Geometry: see drawing. Coordinates: mm, zero at the bounding-box minimum. Give positions to 0.01 mm unless a question says otherwise; leave off trailing zeros. Write each loop counter-clockwise with the first axis right and the second up, starting at its lowest first coordinate (ties: lowest second). Pieces come first, ordered by that corner, then holes. Notation, with made-up numbers: (-16, -25) -> (32, -25) arc R23 cw to (32, -12) -> close; hole circle Ø7 at (-5.5, 26). An arc over 180 degrees is marked (long way). Use one line per item in the form item = value. Start each with the question number.
(1) Material intervals for line 1 along X through (y, z) = (1.8, 59) (3 decimals); line 2 along X through (y, z) = (1.25, 22.75) (3 decimals); line 3 along Z through (x, y) = (9, 1.5), sorted ascending. Write a range as from..to.
(2) First-contact query: P1, Ø2.5, axis at x = 28, z = 59, coming from the -Y side. Flat tip, straight axial feed; report the tip coordinate or a pass-through.
(3) Cut plane A-A, the plane x = 42. Output: boundary loops of the cut face in (y, z) (3 decimals), and give its area (3 significant figures).
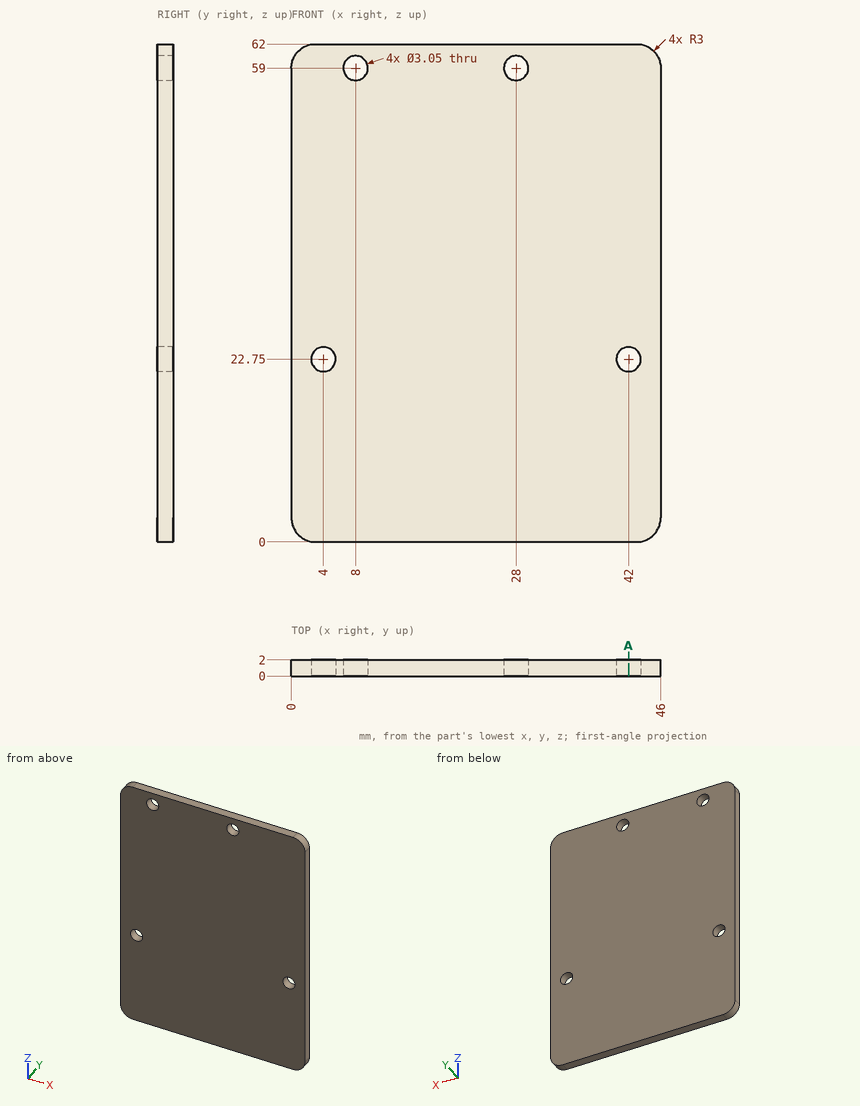
Geometry says:
q1.line_1 = 0..6.475, 9.525..26.475, 29.525..46
q1.line_2 = 0..2.475, 5.525..40.475, 43.525..46
q1.line_3 = 0..57.85, 60.15..62
q2.P1 = through
q3.outline = (0, 0) -> (2, 0) -> (2, 21.225) -> (0, 21.225) -> close; (0, 24.275) -> (2, 24.275) -> (2, 62) -> (0, 62) -> close
q3.area = 118 mm^2
